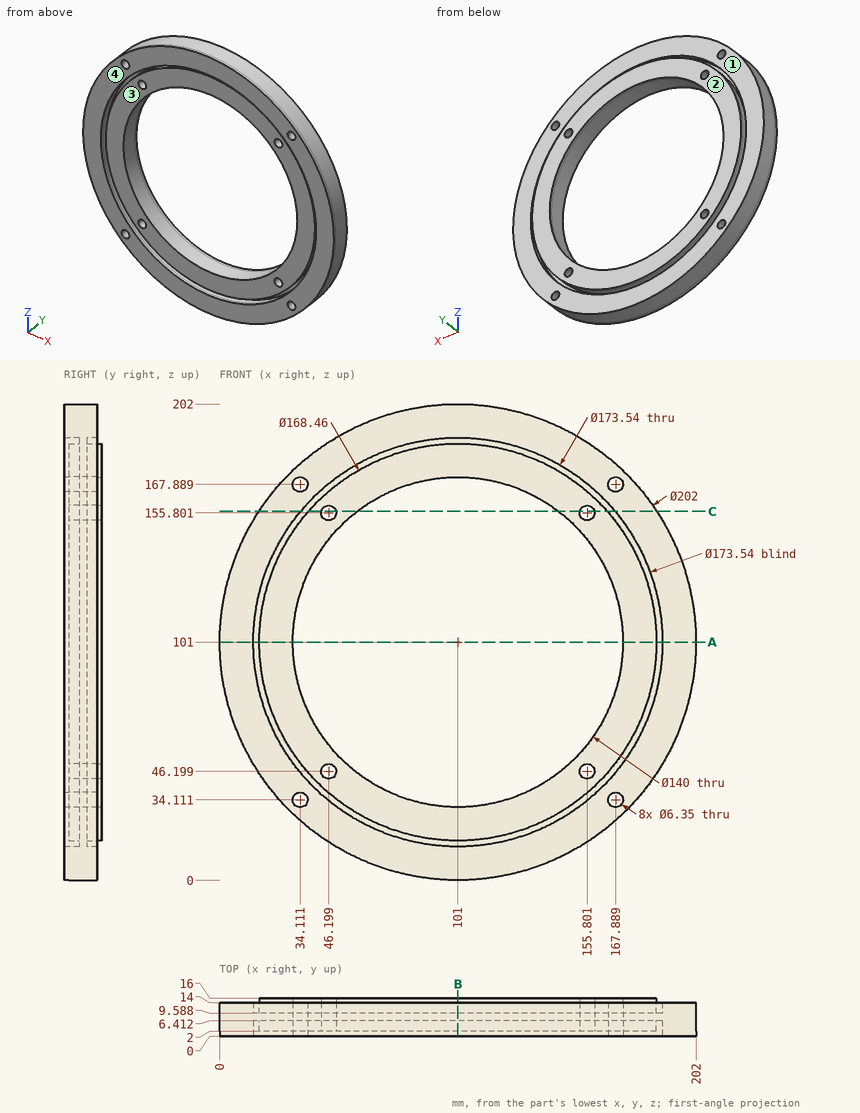
Design review of the part shown in the three views and the two pictorial views. Dimensions are in mm from the part's minimum x, y and z. A direction names the side the tool comes from. Give positions to 0.01 mm unless a question says otherwise; leave off trailing zeros. Loops run counter-clockwise (first coordinate to the right, second up) from the corner with the lowest first, then second, coordinate; pieces in that order, holes last. Notation, with made-up numbers: (6, 46.25) -> (51, 46.25) arc R26 ccw to (51, 63.25) -> close; hole circle Ø3 at (-22.5, 19). An arc over 180 degrees is marked (long way). One line per item, written item: value.
Q1. For pin 1 Ø4 at (y, z) = (8, 40) entering from +X (1 decimal); pin 2 Ø8.5 at (x, z) = (167.89, 34.11) entering from +Y; pin 3 Ø3 at (x, z) = (165, 59.5) entering from -Y, all flat-tipped, find the tip position at first contact; note any pin that passes through.
Numbers:
pin 1: stops at x = 183
pin 2: stops at y = 14
pin 3: stops at y = 2
Q2. We need section A-A on z = 101. Give the boundary of the cut face in (x, y), and give its area (3 significant figures).
Numbers:
outline: (0, 0) -> (14.23, 0) -> (14.23, 6.41) -> (16.77, 6.41) -> (16.77, 2) -> (31, 2) -> (31, 16) -> (16.77, 16) -> (16.77, 9.59) -> (14.23, 9.59) -> (14.23, 14) -> (0, 14) -> close; (171, 2) -> (185.23, 2) -> (185.23, 6.41) -> (187.77, 6.41) -> (187.77, 0) -> (202, 0) -> (202, 14) -> (187.77, 14) -> (187.77, 9.59) -> (185.23, 9.59) -> (185.23, 16) -> (171, 16) -> close
area: 813 mm^2
Q3. Machinability: for the marked faces 1 and 2, which of the approach directions +Z, -Z, +X, -X, +Y, -Y give a long, thin tool a straight path to every point of the face, cutting with its end or side? Answer none if there is none.
Numbers:
face 1: +Y
face 2: +Z, -Z, +X, -X, +Y
Q4. We need section B-B on x = 101. Give the boundary of the cut face in (y, z).
Numbers:
outline: (0, 0) -> (14, 0) -> (14, 14.23) -> (9.59, 14.23) -> (9.59, 16.77) -> (16, 16.77) -> (16, 31) -> (2, 31) -> (2, 16.77) -> (6.41, 16.77) -> (6.41, 14.23) -> (0, 14.23) -> close; (0, 187.77) -> (6.41, 187.77) -> (6.41, 185.23) -> (2, 185.23) -> (2, 171) -> (16, 171) -> (16, 185.23) -> (9.59, 185.23) -> (9.59, 187.77) -> (14, 187.77) -> (14, 202) -> (0, 202) -> close
Q5. For L1, parallel to Z at x = 122, y = 4.75 (1 decimal); L2, parallel to Z at x = 54, y = 13.5 (1 decimal); L3, parallel to X at y = 10.75, z = 158 (1 decimal), list the stretches that pass through material, from the lowest coordinate up.
Numbers:
L1: z = 2.2 to 16.8, 19.4 to 34.2, 167.8 to 182.6, 185.2 to 199.8
L2: z = 11.6 to 28.1, 31.1 to 49.1, 152.9 to 170.9, 173.9 to 190.4
L3: x = 17.6 to 35.6, 39 to 43.9, 48.5 to 60.4, 141.6 to 153.5, 158.1 to 163, 166.4 to 184.4
Q6. Draft analysis for pull direction X (two halves, no side actions). For the marked faces 3 and 4, state which applies: pulls with the +X half, pulls with the -X half, needs draft (parallel to the pull), parting line crosses it, or undercut.
Numbers:
face 3: undercut
face 4: needs draft
Q7. We need section C-C on z = 156.5. Give the number of separate pieces and of enclosed holes in the cut face.
Numbers:
separate pieces: 4
enclosed holes: 0
